Part print with two shaded views. Sizes in mm from the minimum x, y, z corner. Give positions to 0.01 mm unless a question says otherwise; leave off trailing zeros. Loops run counter-clockwise (first coordinate to the right, second up) from the corner with the lowest first, then second, coordinate; pieces in that order, holes last. Notation, with made-up numbers: M 40.5,30 L 75.5,30 A11 cw 75.5,40 Z; hole C 21,-21 d2. An arc over 180 degrees is marked long. Answer as a JSON object with one key per item and string values. Group by question number.
1. Slice it at D-D (z = 16). List the corners of the cut face in (x, y).
2. Drop flat-ended pins along their axis: pin 1 Ø5 at (x, z) = (12.5, 31) entering from +Y; pin 2 Ø1 at (x, z) = (26.5, 34) entering from +Y; pin 3 Ø2 at (x, z) = (18, 18) entering from -Y. Give the stop position or say it passes through.
3. Mould opens along Y. For the marked faces 1, 2 and 3 say: released by +Y, released by -Y, zero draft, split by the parting line, or undercut.
4. Drill centre lines: line 1 along X through (y, z) = (19, 39); line 2 along X through (y, z) = (19, 52). Where is each one in solid material? Low to high. Write a range as [from, to].
5. Slice it at C-C (y = 14.5). List the corners of the cut face in (x, z).
6. Slice it at A-A (y = 19.05). List the corners of the cut face in (x, z).
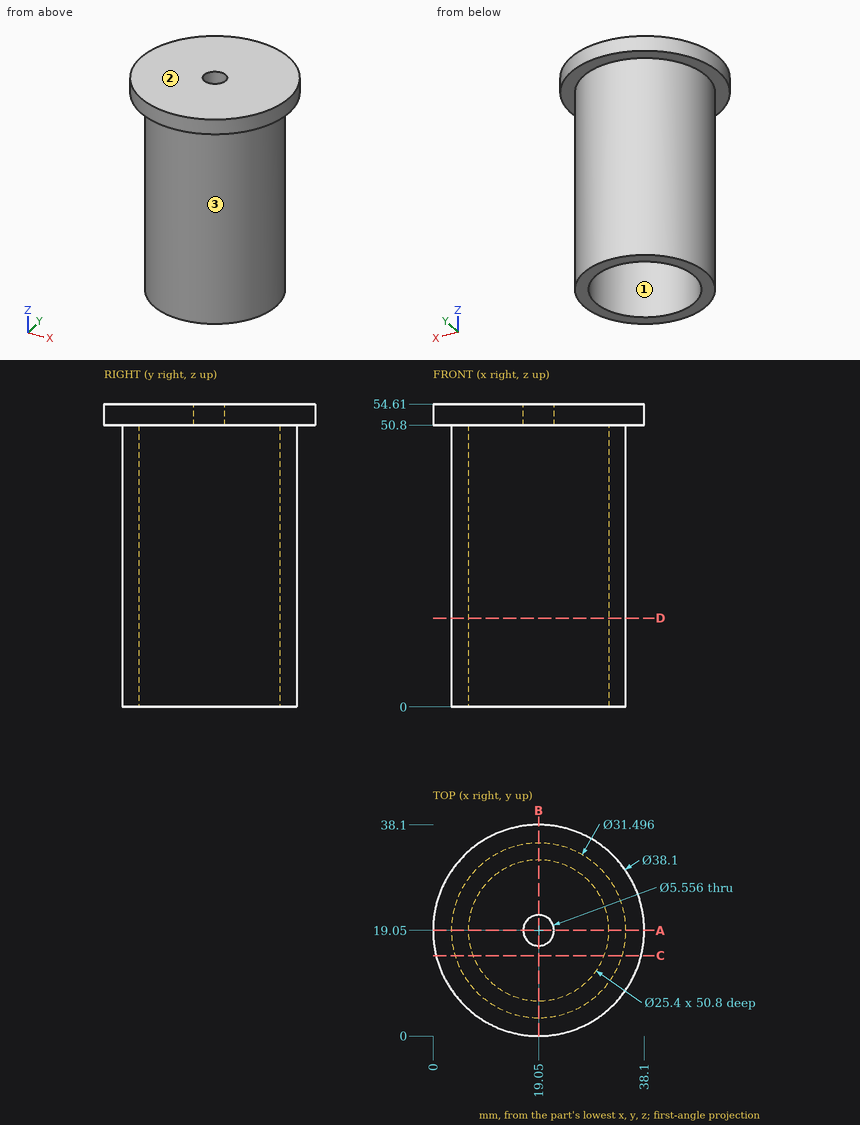
Established:
{
 "1": {"outline": "C 19.05,19.05 d31.5; hole C 19.05,19.05 d25.4"},
 "2": {"pin 1": "stops at y = 34.27", "pin 2": "stops at y = 33.18", "pin 3": "stops at y = 3.3"},
 "3": {"face 1": "undercut", "face 2": "zero draft", "face 3": "split by the parting line"},
 "4": {"line 1": "x = [3.3, 6.35], [31.75, 34.8]", "line 2": "x = [0, 16.27], [21.83, 38.1]"},
 "5": {"outline": "M 0.55,50.8 L 3.97,50.8 L 3.97,0 L 7.19,0 L 7.19,50.8 L 30.91,50.8 L 30.91,0 L 34.13,0 L 34.13,50.8 L 37.55,50.8 L 37.55,54.61 L 0.55,54.61 Z"},
 "6": {"outline": "M 0,50.8 L 3.3,50.8 L 3.3,0 L 6.35,0 L 6.35,50.8 L 16.27,50.8 L 16.27,54.61 L 0,54.61 Z; M 21.83,50.8 L 31.75,50.8 L 31.75,0 L 34.8,0 L 34.8,50.8 L 38.1,50.8 L 38.1,54.61 L 21.83,54.61 Z"}
}
